```python
from build123d import *

# Parameters (mm, degrees)
SKETCH1_W           = 59.88
SKETCH1_H           = 59.88
BOSS_EXTRUDE1_DEPTH = 59.88
CUT_EXTRUDE1_DEPTH  = 30
SKETCH4_R           = 6
BOSS_EXTRUDE3_DEPTH = 10
BOSS_EXTRUDE4_DEPTH = 10


with BuildPart() as part:
    # Sketch1 → Boss-Extrude1 (new body)
    with BuildSketch(Plane(origin=(0, 0, 0), x_dir=(1, 0, 0), z_dir=(0, 1, 0))):
        with Locations((-10.472375433, -22.138876894)):
            Rectangle(SKETCH1_W, SKETCH1_H)
    extrude(amount=BOSS_EXTRUDE1_DEPTH)

    # Sketch2 → Cut-Extrude1 (cut)
    with BuildSketch(Plane.XZ):
        Polygon((-10.472375433, 2.168876894), (-10.472375433, 7.168876894), (-10.472375433, 12.168876894), (-11.972375433, 12.168876894), (-11.972375433, 2.168876894), align=None)
        Polygon((-10.472375433, 12.168876894), (-10.472375433, 7.168876894), (-10.472375433, 2.168876894), (-8.972375433, 2.168876894), (-8.972375433, 12.168876894), align=None)
        Polygon((-8.972375433, 32.108876894), (-10.472375433, 32.108876894), (-11.972375433, 32.108876894), (-11.972375433, 42.108876894), (-8.972375433, 42.108876894), align=None)
    extrude(amount=-CUT_EXTRUDE1_DEPTH, mode=Mode.SUBTRACT)

    # Sketch4 → Boss-Extrude3 (add)
    with BuildSketch(Plane.ZY.offset(40.412375433)):
        with Locations(Location((7.168876894, 44.91, 0), (0, 0, 180))):
            Circle(SKETCH4_R)
        with Locations(Location((37.108876894, 44.91, 0), (0, 0, 180))):
            Circle(SKETCH4_R)
    extrude(amount=BOSS_EXTRUDE3_DEPTH)

    # Sketch5 → Boss-Extrude4 (add)
    with BuildSketch(Plane.ZY.offset(40.412375433)):
        Polygon((20.138876894, 21.94), (20.138876894, 35.94), (24.138876894, 35.94), (24.138876894, 29.94), (24.138876894, 21.94), align=None)
        with BuildLine():
            Line((11.199558119, 15.032847323), (32.61038324, 15.032847323))
            add(Edge.make_bspline(
                [(11.199558119, 15.032847323), (22.018966273, 2.880785428), (32.61038324, 15.032847323)],
                knots=[0, 0, 0, 1, 1, 1], degree=2))
        make_face()
    extrude(amount=BOSS_EXTRUDE4_DEPTH)


solid = part.part
```
Work out the finished part from the listing and answer in its coordinate system (mm). A direction names the side the tool comes from. Coordinates: 2 decimals unless noted, no trailing zeros. Order: outer loops, then holes, each group sorted by start corner. A loop starts at its lowest first (then second) coordinate and runs counter-clockwise, first axis right, second up. Notation, with made-up numbers: (31.5, 22.25) - (87.5, 22.25) arc R23 cw to (87.5, 35.25) - close; hole circle Ø11 at (17.5, 67). An arc over 180 degrees is marked (long way). Answer as a JSON object with one key per item and string values.
1. Find section B-B on x = -41.5. Count the separate pieces of the cut face and the enclosed holes in it, plus the area to 3 significant figures.
Output values:
{"separate pieces": "4", "enclosed holes": "0", "area": "369 mm²"}
2. Find section A-A on y = 32. Determine the outline of the cut face in (x, z), plus the area to 3 significant figures.
Output values:
{"outline": "(-50.41, 20.14) - (-40.41, 20.14) - (-40.41, -7.8) - (19.47, -7.8) - (19.47, 52.08) - (-40.41, 52.08) - (-40.41, 24.14) - (-50.41, 24.14) - close", "area": "3,630 mm²"}
3. Each of these flat-tipped pins is pushed along its axis until it touches: P1, Ø5, axis at x = -45, y = 27, coming from the +Z side; P2, Ø5, axis at y = 12.5, z = 39, coming from the -X side; P3, Ø3, axis at x = -45.5, y = 25.5, coming from the -Z side; P4, Ø11, axis at x = -43, z = 26.5, coming from the +Y side. Where does it stop, or does it pass through?
Output values:
{"P1": "stops at z = 24.14", "P2": "stops at x = -40.41", "P3": "stops at z = 20.14", "P4": "stops at y = 59.88"}
4. A tool of negligible diameter and unlimited length cuts with its end or side. For faces 4 (the face through (-45, 29, 24.139)), 5 (the face through (-45, 21.94, 22)), 6 (the face through (-10, 30, 37)), from which of +Z, -Z, +X, -X, +Y, -Y can it reach the whole face along a straight path? Write none if from no direction.
Output values:
{"face 4": "+Z, -X, +Y", "face 5": "+Z, -Z, -X", "face 6": "-Y"}
5. Find section C-C on y = 44.91. Determine the outline of the cut face in (x, z), plus the area to 3 significant figures.
Output values:
{"outline": "(-50.41, 1.17) - (-40.41, 1.17) - (-40.41, -7.8) - (19.47, -7.8) - (19.47, 52.08) - (-40.41, 52.08) - (-40.41, 43.11) - (-50.41, 43.11) - (-50.41, 31.11) - (-40.41, 31.11) - (-40.41, 13.17) - (-50.41, 13.17) - close", "area": "3,830 mm²"}
6. The mould has two halves that part along X. Classify faces 1 (the face through (-50.412, 12, 22)), 2 (the face through (-11, 0, 22)), 3 (the face through (-8.972, 15, 7)): +X half, -X half, draft (parallel to the pull), parting line (faces both ways), or undercut.
Output values:
{"face 1": "-X half", "face 2": "draft", "face 3": "undercut"}
7. Consider line 1 (X direction, y = 47.5, z = 48.5); line 2 (Y direction, x = -46, z = 24); line 3 (Z direction, x = -41.5, y = 26.5). Determine where each line is inside the solid, lowest interval first.
Output values:
{"line 1": "x = -40.41 to 19.47", "line 2": "y = 9.18 to 15.03, 21.94 to 35.94", "line 3": "z = 20.14 to 24.14"}
